Source: three-view drawing plus pictorial views. Frame: mm from the lowest corner of the part. A direction names the side the tool comes from. Round coordinates to 2 decimals unless told otherwise and drop trailing zeros. Loops run counter-clockwise (first coordinate to the right, second up) from the corner with the lowest first, then second, coordinate; pieces in that order, holes last. Notation, with made-up numbers: M -34,71.5 L 14,71.5 A35 ccw 14,106.5 Z; hole C 44,-17.5 d4. An arc over 180 degrees is marked long. Write each question's results on one line, items separated by ' | '.
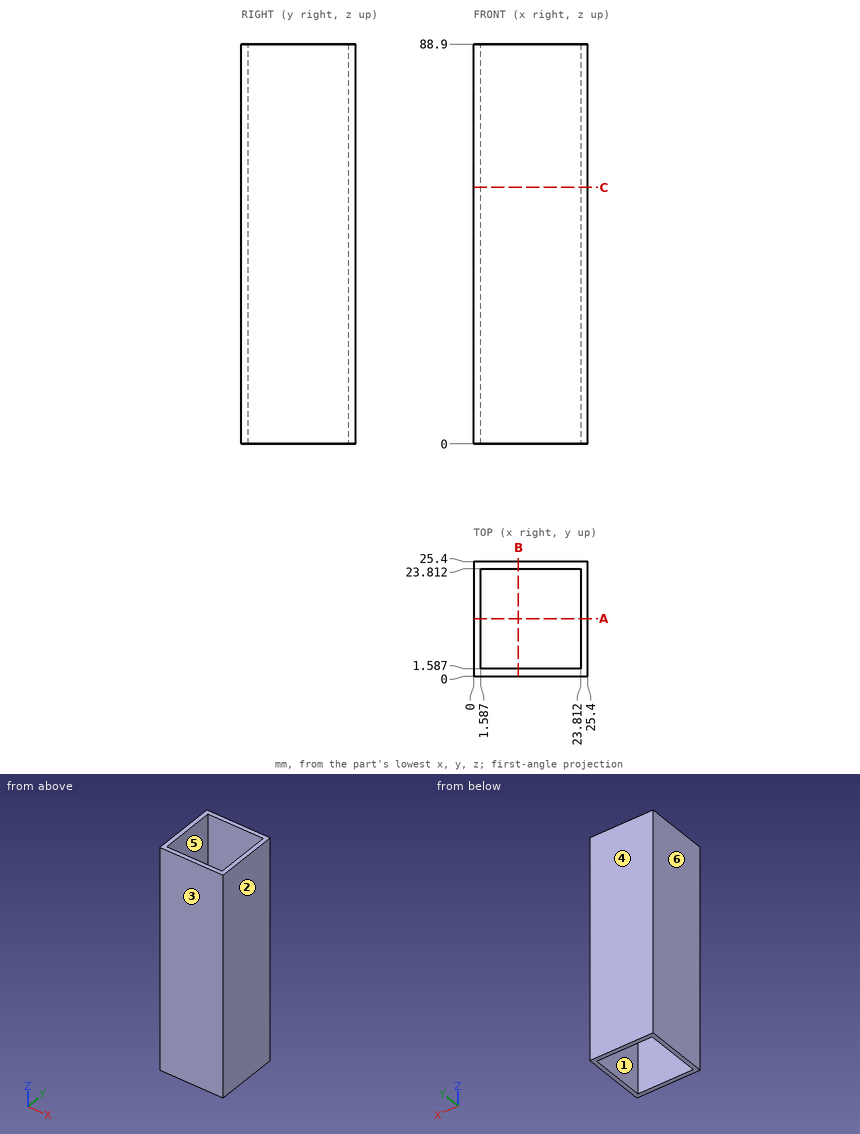
1. Section A-A (y = 12.75). Output: boundary loops of the cut face in (x, z).
Answer key:
outline: M 0,0 L 1.59,0 L 1.59,88.9 L 0,88.9 Z; M 23.81,0 L 25.4,0 L 25.4,88.9 L 23.81,88.9 Z
2. Section C-C (z = 57). Output: boundary loops of the cut face in (x, y).
Answer key:
outline: M 0,0 L 25.4,0 L 25.4,25.4 L 0,25.4 Z; hole M 1.59,1.59 L 23.81,1.59 L 23.81,23.81 L 1.59,23.81 Z
3. Pin query (flat end, axial travel): P1, Ø6, axis at y = 10, z = 67.5, coming from the -X side. Return the tip coordinate at first contact, or that it passes through.
Answer key:
P1: stops at x = 0
4. Ray query, probe 1 along Y at (x, z) = (16, 66). Return the intervals inside material, ascending.
Answer key:
probe 1: y = 0 to 1.59, 23.81 to 25.4
5. Access query for the marked faces 1 and 2. Directions: +Z, -Z, +X, -X, +Y, -Y. A direction counts if a zero-diameter tool reaches every point of the face in a straight line with its end or side. Return the directions, or none.
Answer key:
face 1: +Z, -Z | face 2: +Z, -Z, +X, +Y, -Y
6. Draft query along Y for the marked faces 3, 4, 5 and 6. Return one class per face: pulls with the +Y half, pulls with the -Y half, needs draft (parallel to the pull), parting line crosses it, or undercut.
Answer key:
face 3: pulls with the -Y half | face 4: pulls with the +Y half | face 5: undercut | face 6: needs draft
